Could you check a few things on this model? Use its own coordinates, in mm. Face numbers are marked on the shaded views. A direction names the side the tool comes from. Round coordinates to 2 decimals unless told otherwise and drop trailing zeros. Write each loop counter-clockwise with the first axis right and the second up, starting at its lowest first coordinate (ties: lowest second). Pieces come first, ordered by that corner, then holes. Notation, with made-up numbers: M 45.5,-15.75 L 73.5,-15.75 A31 ccw 73.5,16.25 Z; hole C 17,-17.5 d3. An arc over 180 degrees is marked long. One line per question, with ' | ' between items. Start each with the question number.
```python
from build123d import *

# Parameters (mm, degrees)
SKETCH2_W           = 155
SKETCH2_H           = 80
BOSS_EXTRUDE1_DEPTH = 15
SKETCH3_W           = 15
SKETCH3_H           = 70
CUT_EXTRUDE1_DEPTH  = 5
SKETCH4_W           = 155
SKETCH4_H           = 80
BOSS_EXTRUDE3_DEPTH = 60
SKETCH5_W           = 155
SKETCH5_H           = 80
SKETCH5_W_2         = 149
SKETCH5_H_2         = 74
CUT_EXTRUDE2_DEPTH  = 3
FILLET1_R           = 2


with BuildPart() as part:
    # Sketch2 → Boss-Extrude1 (new body)
    with BuildSketch(Plane(origin=(0, 0, 0), x_dir=(1, 0, 0), z_dir=(0, 1, 0))):
        with Locations((-77.5, -40)):
            Rectangle(SKETCH2_W, SKETCH2_H)
    extrude(amount=BOSS_EXTRUDE1_DEPTH)

    # Sketch3 → Cut-Extrude1 (cut)
    with BuildSketch(Plane(origin=(0, 15, 0), x_dir=(1, 0, 0), z_dir=(0, 1, 0))):
        with Locations((-77.5, -40)):
            Rectangle(SKETCH3_W, SKETCH3_H)
    extrude(amount=-CUT_EXTRUDE1_DEPTH, mode=Mode.SUBTRACT)

    # Sketch4 → Boss-Extrude3 (add)
    with BuildSketch(Plane(origin=(0, 15, 0), x_dir=(1, 0, 0), z_dir=(0, 1, 0))):
        with Locations((-77.5, -40)):
            Rectangle(SKETCH4_W, SKETCH4_H)
        Polygon((-145, -10), (-145, -70), (-85, -70), (-85, -75), (-70, -75), (-70, -70), (-10, -70), (-10, -10), (-70, -10), (-70, -5), (-85, -5), (-85, -10), align=None, mode=Mode.SUBTRACT)
    extrude(amount=BOSS_EXTRUDE3_DEPTH)

    # Sketch5 → Cut-Extrude2 (cut)
    with BuildSketch(Plane(origin=(0, 75, 0), x_dir=(1, 0, 0), z_dir=(0, 1, 0))):
        with Locations((-77.5, -40)):
            Rectangle(SKETCH5_W, SKETCH5_H)
        with Locations((-77.5, -40)):
            Rectangle(SKETCH5_W_2, SKETCH5_H_2, mode=Mode.SUBTRACT)
    extrude(amount=-CUT_EXTRUDE2_DEPTH, mode=Mode.SUBTRACT)

    # Fillet1
    fillet1_edges = [part.edges().sort_by_distance(p)[0] for p in [
        (-77.5, 0, 80),
        (-155, 0, 40),
        (-77.5, 0, 0),
        (0, 0, 40),
        (0, 36, 0),
        (0, 36, 80),
        (-155, 36, 0),
        (-155, 36, 80),
    ]]
    fillet(fillet1_edges, radius=FILLET1_R)


solid = part.part
```
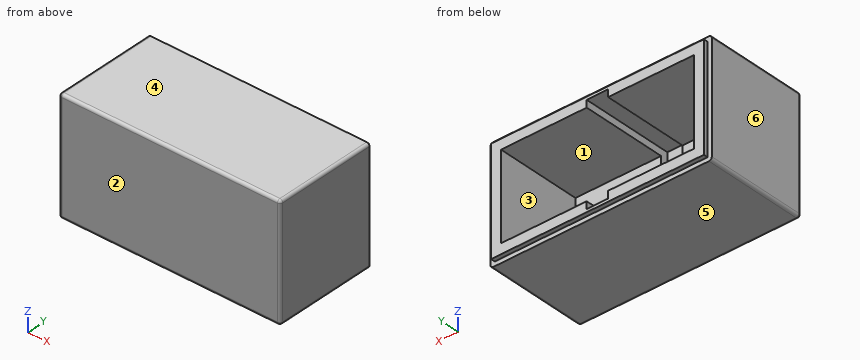
1. Which directions (+Z, -Z, +X, -X, +Y, -Y) give clear straight access to the entire face, cutting with the end or side of a thin tool? Please do the marked faces 1 and 2.
2. I need wall thicknesses on line 1 along X through (y, z) = (69.5, 19); line 2 along Z through (x, y) = (-22, 55.5); line 3 along Y through (x, z) = (-117.5, 25). Which ranges of each line are inside material? Lowest first, please. Write a range as from..to.
3. Suppose I cut it at A-A (y = 60). Write out the boundary of the cut face in (x, z).
4. Suppose I cut it at B-B (z = 57). Write out the boundary of the cut face in (x, y).
5. I'm going to push flat-ended pins straight in: P1, Ø1.5, axis at y = 73.5, z = 38, coming from the +X side; P2, Ø16.5, axis at x = -79.5, z = 34, coming from the +Y side; P3, Ø2.5, axis at x = -76.5, y = 73, coming from the +Z side; P4, Ø1.5, axis at y = 74, z = 54.5, coming from the -X side. Where does each tip first touch, or does it pass through?
6. If we mould it in two halves opening along Z, with no side actions, what happens to the marked faces 3, 4, 5 and 6? For each: released by +Z, released by -Z, zero draft, split by the parting line, or undercut.
7. Suppose I cut it at C-C (x = -128). Write out the boundary of the cut face in (y, z).
Computed:
1) face 1: +Y | face 2: +Z, -Z, +X, -X, -Y
2) line 1: x = -155..-145, -10..0 | line 2: z = 0..10, 70..80 | line 3: y = 0..15
3) outline: M -155,2 A2 ccw -153,0 L -2,0 A2 ccw 0,2 L 0,78 A2 ccw -2,80 L -153,80 A2 ccw -155,78 Z; hole M -145,10 L -85,10 L -85,5 L -70,5 L -70,10 L -10,10 L -10,70 L -70,70 L -70,75 L -85,75 L -85,70 L -145,70 Z
4) outline: M -155,2 A2 ccw -153,0 L -2,0 A2 ccw 0,2 L 0,72 L -3,72 L -3,75 L -10,75 L -10,15 L -70,15 L -70,10 L -85,10 L -85,15 L -145,15 L -145,75 L -152,75 L -152,72 L -155,72 Z
5) P1: stops at x = -3 | P2: stops at y = 15 | P3: stops at z = 80 | P4: stops at x = -152
6) face 3: undercut | face 4: released by +Z | face 5: released by -Z | face 6: zero draft
7) outline: M 0,2 A2 ccw 2,0 L 72,0 L 72,3 L 75,3 L 75,10 L 15,10 L 15,70 L 75,70 L 75,77 L 72,77 L 72,80 L 2,80 A2 ccw 0,78 Z
